Input: dimensioned drawing with shaded views. Units: mm. Origin: part minimum x, y, z. A direction names the side the tool comes from. Round coordinates to 2 decimals unless told otherwise and drop trailing zeros. Loops run counter-clockwise (first coordinate to the right, second up) from the corner with the lowest first, then second, coordinate; pieces in that order, holes last. Notation, with made-up numbers: M 6,38 L 54,38 A27 cw 54,68 Z; hole C 50.5,56.25 d7. An arc over 180 degrees is marked long. Use one line per item in the form item = value. Start each with the question number.
Q1. Section query B-B, the plane y = 13.5. Output: boundary loops of the cut face in (x, z), and give its area (3 significant figures).
Q2. Section query A-A, the plane z = 6.6. Output: boundary loops of the cut face in (x, y) (3 decimals).
Q3. Section query D-D, the plane y = 22.75. Output: boundary loops of the cut face in (x, z), and give its area (3 significant figures).
Q4. First-contact query: P1, Ø5, axis at x = 82.5, z = 7, coming from the -Y side (3 decimals); P2, Ø7.5, axis at y = 13, z = 5.5, coming from the -X side; P3, Ø6, axis at x = 85.5, y = 14.5, coming from the +Z side; P4, Ø5, axis at x = 88, z = 7, coming from the +Y side (3 decimals). Flat tips, straight axial feed; report the tip coordinate or a pass-through.
Q5. Section query C-C, the plane z = 1. Output: boundary loops of the cut face in (x, y).
Q6. Access query for the marked faces 1, 2, 3 and 4. Directions: +Z, -Z, +X, -X, +Y, -Y. A direction counts if a zero-diameter tool reaches every point of the face in a straight line with its end or side. Return the directions, or none.
Q7. Ray query, line 1 along X through (y, z) = (22, 4.25); line 2 along X through (y, z) = (12, 4); line 3 along Y through (x, z) = (85.5, 8.75) (3 decimals). Return the intervals inside material, ascending.
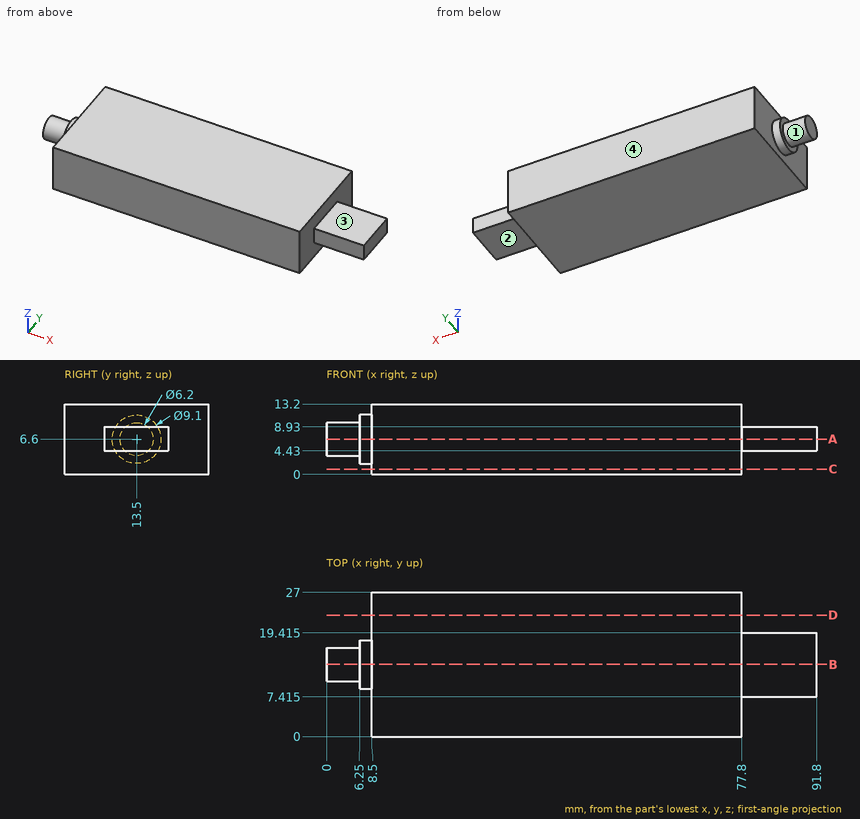
Results found:
q1.outline = M 0,3.5 L 6.25,3.5 L 6.25,2.05 L 8.5,2.05 L 8.5,0 L 77.8,0 L 77.8,4.43 L 91.8,4.43 L 91.8,8.93 L 77.8,8.93 L 77.8,13.2 L 8.5,13.2 L 8.5,11.15 L 6.25,11.15 L 6.25,9.7 L 0,9.7 Z
q1.area = 1,040 mm²
q2.outline = M 0,10.4 L 6.25,10.4 L 6.25,8.95 L 8.5,8.95 L 8.5,0 L 77.8,0 L 77.8,7.415 L 91.8,7.415 L 91.8,19.415 L 77.8,19.415 L 77.8,27 L 8.5,27 L 8.5,18.05 L 6.25,18.05 L 6.25,16.6 L 0,16.6 Z
q3.outline = M 8.5,0 L 77.8,0 L 77.8,13.2 L 8.5,13.2 Z
q3.area = 915 mm²
q4.P1 = 7.415
q4.P2 = 0
q4.P3 = 8.93
q4.P4 = 19.415
q5.outline = M 8.5,0 L 77.8,0 L 77.8,27 L 8.5,27 Z
q6.face_1 = -X
q6.face_2 = -Z, +X, +Y, -Y
q6.face_3 = +Z, +X, +Y, -Y
q6.face_4 = +Z, -Z, +X, -X, +Y
q7.line_1 = 8.5 to 77.8
q7.line_2 = 0 to 77.8
q7.line_3 = 7.415 to 19.415
